The model under review builds one solid part; all positions refer to its coordinate system, in mm. Face numbers are marked on the shaded views. Give positions to 0.01 mm unless a question says otherwise; leave off trailing zeros. Loops run counter-clockwise (first coordinate to the right, second up) from the corner with the lowest first, then second, coordinate; pieces in that order, holes last. Notation, with made-up numbers: (-1.5, 16.25) -> (29.5, 16.25) arc R23 cw to (29.5, 42.25) -> close; hole circle Ø3 at (30, 75). An arc over 180 degrees is marked (long way). Write each question's results on one line, items separated by ' | '. Start each with the question number.
Q1. We need section A-A (z = -8). Write out the cut boundary in (x, y), plus the area to 3 significant figures.
Q2. Insertion check: pin 1 Ø4 at (x, y) = (-43.5, 4.5) entering from -Z; pin 2 Ø8.5 at (x, y) = (-48.82, 15.8) entering from +Z; pin 3 Ø6 at (y, z) = (10.5, -27.5) entering from -X. Each pin has a flat end and moves straight along its axis. Give the tip position at first contact, or say it passes through.
Q3. We need section D-D (x = -37). Write out the cut boundary in (y, z).
Q4. Wall thickness on L1, parallel to X at y = 9, z = -19; L2, parallel to X at y = 6, z = -4; L3, parallel to Z at x = -48.5, y = 23.5: over which ranges is each line inside the solid? List them lowest first. Write a range as [from, to].
Q5. Mouldability with a two-part tool opening along X and no side actions: class the marked faces 1, 2 and 3 as released by +X, released by -X, zero draft, split by the parting line, or undercut.
Q6. We need section B-B (z = -26). Write out the cut boundary in (x, y) (3 decimals).
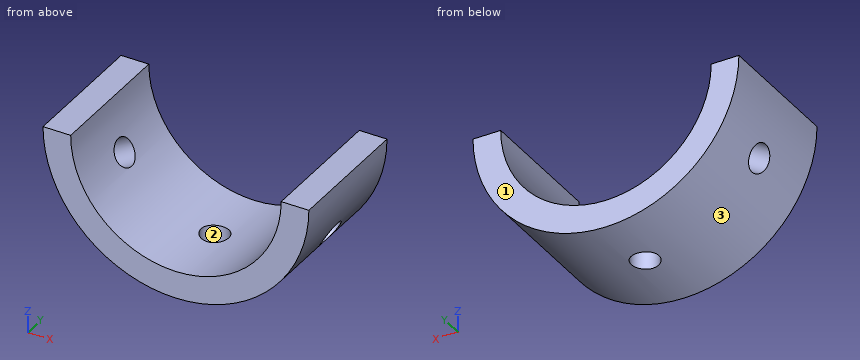
from build123d import *

# Parameters (mm, degrees)
BOSS_EXTRUDE1_DEPTH = 30.48
SKETCH3_R           = 24.13
CUT_EXTRUDE4_DEPTH  = 90.914560616
SKETCH4_R           = 3.175
CUT_EXTRUDE5_DEPTH  = 63.754
CIRPATTERN3_COUNT   = 6


with BuildPart() as part:
    # Sketch1 → Boss-Extrude1 (new body)
    with BuildSketch(Plane(origin=(0, 0, 0), x_dir=(1, 0, 0), z_dir=(0, 1, 0))):
        with BuildLine():
            Line((-78.958715675, 0), (-17.998715675, 0))
            ThreePointArc((-17.998715675, 0), (-48.478715675, 30.349942827), (-78.958715675, 0))
        make_face()
    extrude(amount=BOSS_EXTRUDE1_DEPTH)

    # Sketch3 → Cut-Extrude4 (cut, through all)
    with BuildSketch(Plane(origin=(0, 0, 0), x_dir=(1, 0, 0), z_dir=(0, 1, 0))):
        with Locations((-48.478715675, 0)):
            Circle(SKETCH3_R)
    extrude(amount=CUT_EXTRUDE4_DEPTH, mode=Mode.SUBTRACT)

    # Sketch4 → Cut-Extrude5 (cut)
    with BuildSketch(Plane.XY):
        with Locations((-48.824364134, 15.798935299)):
            Circle(SKETCH4_R)
    cut_extrude5 = extrude(amount=-CUT_EXTRUDE5_DEPTH, mode=Mode.SUBTRACT)

    # CirPattern3: Cut-Extrude5 ×6 about axis
    cirpattern3_axis = Axis((-48.478715675, 30.48, 0.130335837), (0, -1, 0))
    for i in range(1, CIRPATTERN3_COUNT):
        add(cut_extrude5.rotate(cirpattern3_axis, i * 360 / CIRPATTERN3_COUNT), mode=Mode.SUBTRACT)


solid = part.part
Output:
1) outline: (-77.85, 0) -> (-71.24, 0) -> (-71.24, 30.48) -> (-77.85, 30.48) -> close; (-25.71, 0) -> (-19.1, 0) -> (-19.1, 30.48) -> (-25.71, 30.48) -> close | area: 403 mm2
2) pin 1: z = -30.2 | pin 2: z = -23.69 | pin 3: x = -66.43
3) outline: (0, -28.11) -> (30.48, -28.11) -> (30.48, -21.22) -> (0, -21.22) -> close
4) L1: [-72.21, -63.35], [-33.6, -24.75] | L2: [-78.68, -72.27], [-24.68, -18.28] | L3: [-30.35, -24.13]
5) face 1: zero draft | face 2: undercut | face 3: split by the parting line
6) outline: (-64.171, 0) -> (-32.786, 0) -> (-32.786, 30.48) -> (-64.171, 30.48) -> close; hole circle Ø6.35 at (-48.824, 15.799)
